Geometry check sheet. Reference: the model listing, model coordinates, mm. Face numbers are marked on the shaded views. A direction names the side the tool comes from. Coordinates: 2 decimals unless noted, no trailing zeros. Loops run counter-clockwise (first coordinate to the right, second up) from the corner with the lowest first, then second, coordinate; pieces in that order, holes last.
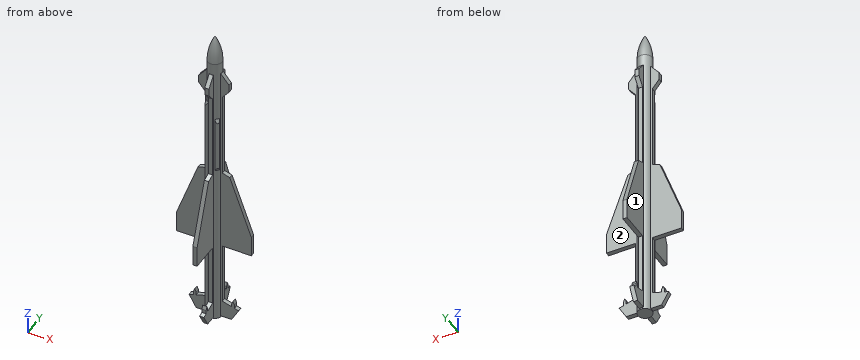
from build123d import *

# Parameters (mm, degrees)
F4_DEPTH  = 0.1
F5_COUNT  = 4
F8_DEPTH  = 10.8333333333
F11_DEPTH = 2.4
F12_SIZE2 = 0.09999
F12_SIZE  = 0.173195


# Not quite as in the source:
# - a fillet or chamfer is up to 0.001 mm smaller than in the source, because OpenCascade refuses the exact size


with BuildPart() as f2:
    # F1 (on Front) → F2 (revolve)
    with BuildSketch(Plane.XZ):
        with BuildLine():
            Line((0, 14.8666666667), (0, 0))
            Line((0, 0), (0.3333333333, 0))
            Line((0.3333333333, 0), (0.3333333333, 13.6))
            ThreePointArc((0.3333333333, 13.6), (0.2486051426, 14.2548960901), (0, 14.8666666667))
        make_face()
    revolve(axis=Axis((0, 0, 7.4333333333), (0, 0, 1)))

    # F3 (on Front) → F4 (join, symmetric)
    with BuildSketch(Plane.XZ):
        Polygon((0, 13.4391304348), (0, 0.0666666667), (0.8333333333, 0.0666666667), (1.1666666667, 0.65), (0.9666666667, 0.71), (0.8333333333, 0.75), (0.4, 0.88), (0.4, 3.8333333333), (1.7666666667, 3.8333333333), (1.7666666667, 4.8166666667), (0.75, 7.6333333333), (0.4, 7.7453333333), (0.4, 11.8144927536), (0.7166666667, 12.2), (0.7166666667, 12.5666666667), align=None)
        Polygon((0.8333333333, 0.75), (0.9666666667, 0.71), (0.9666666667, 0.8890524292), (0.9, 1.05), (0.8333333333, 0.8890524292), align=None)
    extrude(amount=F4_DEPTH, both=True)

    # F5: F2 ×4 about axis
    f5_axis = Axis((0, 0, 0), (0, 0, 1))


with BuildPart() as f2_1:
    add(f2.part)
    for i in range(1, F5_COUNT):
        add(f2.part.rotate(f5_axis, i * 360 / F5_COUNT))

    # F7 (on offset) → F8 (join)
    with BuildSketch(Plane.XY.offset(0.4666666667)):
        with BuildLine():
            Line((-0.1110620592, 0.030359297), (-0.3064129385, -0.1649915823))
            ThreePointArc((-0.3064129385, -0.1649915823), (-0.3064129385, -0.3064129385), (-0.1649915823, -0.3064129385))
            Line((-0.1649915823, -0.3064129385), (0.030359297, -0.1110620592))
            Line((0.030359297, -0.1110620592), (-0.1110620592, 0.030359297))
        make_face()
    extrude(amount=F8_DEPTH)

    # F10 (on offset) → F11 (join)
    with BuildSketch(Plane.XY.offset(8.1)):
        with BuildLine():
            Line((0.1737662231, -0.0323448669), (0.0323448669, -0.1737662231))
            Line((0.0323448669, -0.1737662231), (0.1649915823, -0.3064129385))
            ThreePointArc((0.1649915823, -0.3064129385), (0.3064129385, -0.3064129385), (0.3064129385, -0.1649915823))
            Line((0.3064129385, -0.1649915823), (0.1737662231, -0.0323448669))
        make_face()
    extrude(amount=F11_DEPTH)

    # F12 (call 1 of 4: OpenCascade refuses the feature's edges together) (size 0.1732050808 and 0.1 in the source; OpenCascade refuses exactly that, so slightly less here)
    f12_edges = [f2_1.edges().sort_by_distance(p)[0] for p in [
        (-0.235702, -0.235702, 11.3),
    ]]
    f12_side = f2_1.faces().sort_by_distance((-0.333333, 0, 0.013633))[0]
    chamfer(f12_edges, length=F12_SIZE, length2=F12_SIZE2, reference=f12_side)

    # F12#2 (call 2 of 4) (size 0.1732050808 and 0.1 in the source; OpenCascade refuses exactly that, so slightly less here)
    f12_2_edges = [f2_1.edges().sort_by_distance(p)[0] for p in [
        (-0.235702, -0.235702, 0.466667),
    ]]
    f12_2_side = f2_1.faces().sort_by_distance((-0.333333, 0, 0.013633))[0]
    chamfer(f12_2_edges, length=F12_SIZE, length2=F12_SIZE2, reference=f12_2_side)

    # F12#3 (call 3 of 4) (size 0.1732050808 and 0.1 in the source; OpenCascade refuses exactly that, so slightly less here)
    f12_3_edges = [f2_1.edges().sort_by_distance(p)[0] for p in [
        (0.235702, -0.235702, 8.1),
    ]]
    f12_3_side = f2_1.faces().sort_by_distance((-0.333333, 0, 0.013633))[0]
    chamfer(f12_3_edges, length=F12_SIZE, length2=F12_SIZE2, reference=f12_3_side)

    # F12#4 (call 4 of 4) (size 0.1732050808 and 0.1 in the source; OpenCascade refuses exactly that, so slightly less here)
    f12_4_edges = [f2_1.edges().sort_by_distance(p)[0] for p in [
        (0.235702, -0.235702, 10.5),
    ]]
    f12_4_side = f2_1.faces().sort_by_distance((-0.333333, 0, 0.013633))[0]
    chamfer(f12_4_edges, length=F12_SIZE, length2=F12_SIZE2, reference=f12_4_side)


solid = f2_1.part
1) Depth check by flat-ended pin: pin 1 (2 mm diameter, centred on y = 0, z = 7, fed in from -X). Enter the tip coordinate at first touch or a pass-through.
Data:
pin 1: stops at x = -1.34
2) Section check A-A on z = 8.5. Record the cut outline in (x, y) (3 decimals).
Data:
outline: (-0.4, -0.1) - (-0.318, -0.1) arc R0.333 ccw to (-0.296, -0.154) - (-0.306, -0.165) arc R0.1 ccw to (-0.165, -0.306) - (-0.154, -0.296) arc R0.333 ccw to (-0.1, -0.318) - (-0.1, -0.4) - (0.1, -0.4) - (0.1, -0.318) arc R0.333 ccw to (0.154, -0.296) - (0.165, -0.306) arc R0.1 ccw to (0.306, -0.165) - (0.296, -0.154) arc R0.333 ccw to (0.318, -0.1) - (0.4, -0.1) - (0.4, 0.1) - (0.318, 0.1) arc R0.333 ccw to (0.1, 0.318) - (0.1, 0.4) - (-0.1, 0.4) - (-0.1, 0.318) arc R0.333 ccw to (-0.318, 0.1) - (-0.4, 0.1) - close
3) Material ranges on probe 1 along Z at (x, y) = (0.45, -0.05) (3 decimals); probe 2 along Z at (x, y) = (0, 0.6); probe 3 along X at (y, z) = (-0.4, 4.75), recorded low to high.
Data:
probe 1: z = 0.067 to 0.865, 3.833 to 7.729, 11.875 to 12.891
probe 2: z = 0.07 to 0.82, 3.83 to 7.68, 12.06 to 12.71
probe 3: x = -0.1 to 0.1
4) Section check D-D on x = -1.3. Record the cut outline in (y, z).
Data:
outline: (-0.1, 3.83) - (0.1, 3.83) - (0.1, 6.11) - (-0.1, 6.11) - close
5) Section check C-C on y = 1.4. Record the cut outline in (x, z).
Data:
outline: (-0.1, 3.83) - (0.1, 3.83) - (0.1, 5.83) - (-0.1, 5.83) - close
6) Access from +Z, -Z, +X, -X, +Y, -Y to the whole of each face (thin tool, end or side, straight path). Record for the marked faces 1 and 2.
Data:
face 1: +Z, -Z, -X, +Y
face 2: +Z, -Z, +X, +Y
7) Section check B-B on z = 3. Record the cut outline in (x, y) (3 decimals).
Data:
outline: (-0.4, -0.1) - (-0.318, -0.1) arc R0.333 ccw to (-0.296, -0.154) - (-0.306, -0.165) arc R0.1 ccw to (-0.165, -0.306) - (-0.154, -0.296) arc R0.333 ccw to (-0.1, -0.318) - (-0.1, -0.4) - (0.1, -0.4) - (0.1, -0.318) arc R0.333 ccw to (0.318, -0.1) - (0.4, -0.1) - (0.4, 0.1) - (0.318, 0.1) arc R0.333 ccw to (0.1, 0.318) - (0.1, 0.4) - (-0.1, 0.4) - (-0.1, 0.318) arc R0.333 ccw to (-0.318, 0.1) - (-0.4, 0.1) - close
